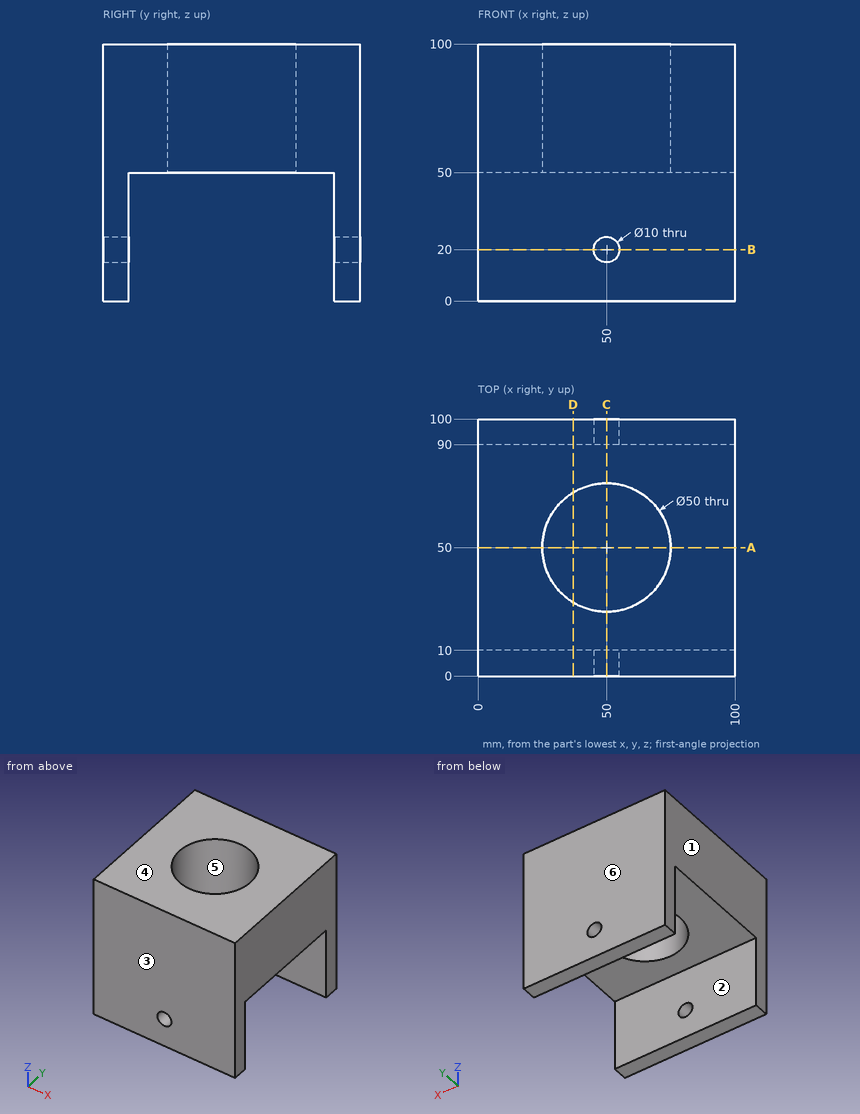
Geometry: see drawing. Coordinates: mm, zero at the bounding-box minimum. A direction names the side the tool comes from. Give positions to 0.01 mm unless a question says otherwise; leave off trailing zeros. Order: outer loops, then holes, each group sorted by start corner. A loop starts at its lowest first (then second) coordinate and runs counter-clockwise, first axis right, second up.
1. Line query: probe 1 along X at (y, z) = (50, 75); probe 2 along Y at (x, z) = (80, 32); probe 3 along Z at (x, y) = (50, 98). Output: solid intervals per line, ascending.
Computed:
probe 1: x = 0 to 25, 75 to 100
probe 2: y = 0 to 10, 90 to 100
probe 3: z = 0 to 15, 25 to 100
2. Set-up query: the marked faces 1 and 2. Return all of +Z, -Z, +X, -X, +Y, -Y with unobstructed straight access to the full face (end or side cutting, diameter ignored); none if empty.
Computed:
face 1: +Z, -Z, -X, +Y, -Y
face 2: -Z, +X, -X
3. Cut plane C-C (x = 50). Return loops of the section in (y, z).
Computed:
outline: (0, 0) - (10, 0) - (10, 15) - (0, 15) - close; (0, 25) - (10, 25) - (10, 50) - (25, 50) - (25, 100) - (0, 100) - close; (75, 50) - (90, 50) - (90, 25) - (100, 25) - (100, 100) - (75, 100) - close; (90, 0) - (100, 0) - (100, 15) - (90, 15) - close
4. Draft query along Y for the marked faces 3, 4, 5 and 6. Return one class per face: released by +Y, released by -Y, zero draft, split by the parting line, or undercut.
Computed:
face 3: released by -Y
face 4: zero draft
face 5: undercut
face 6: released by +Y
5. Cut plane B-B (z = 20). Return loops of the section in (x, y).
Computed:
outline: (0, 0) - (45, 0) - (45, 10) - (0, 10) - close; (0, 90) - (45, 90) - (45, 100) - (0, 100) - close; (55, 0) - (100, 0) - (100, 10) - (55, 10) - close; (55, 90) - (100, 90) - (100, 100) - (55, 100) - close
6. Cut plane D-D (x = 37). Return loops of the section in (y, z), and give its area (3 significant figures).
Computed:
outline: (0, 0) - (10, 0) - (10, 50) - (28.65, 50) - (28.65, 100) - (0, 100) - close; (71.35, 50) - (90, 50) - (90, 0) - (100, 0) - (100, 100) - (71.35, 100) - close
area: 3,860 mm2
7. Cut plane A-A (y = 50). Return loops of the section in (x, z), and give its area (3 significant figures).
Computed:
outline: (0, 50) - (25, 50) - (25, 100) - (0, 100) - close; (75, 50) - (100, 50) - (100, 100) - (75, 100) - close
area: 2,500 mm2
8. Pin query (flat end, axial travel): pin 1 Ø5 at (x, y) = (27.5, 62.5) entering from -Z. Return the tip coordinate at first contact, or that it passes through.
Computed:
pin 1: stops at z = 50
